Source: three-view drawing plus pictorial views. Frame: mm from the lowest corner of the part. A direction names the side the tool comes from. Coordinates: 2 decimals unless noted, no trailing zeros. Order: outer loops, then holes, each group sorted by start corner. A loop starts at its lowest first (then second) coordinate and runs counter-clockwise, first axis right, second up. Notation, with made-up numbers: M -27,35 L -18,35 A15 ccw -18,61 Z; hole C 8,31 d2. An arc over 180 degrees is marked long. One line per question, with ' | ' between items.
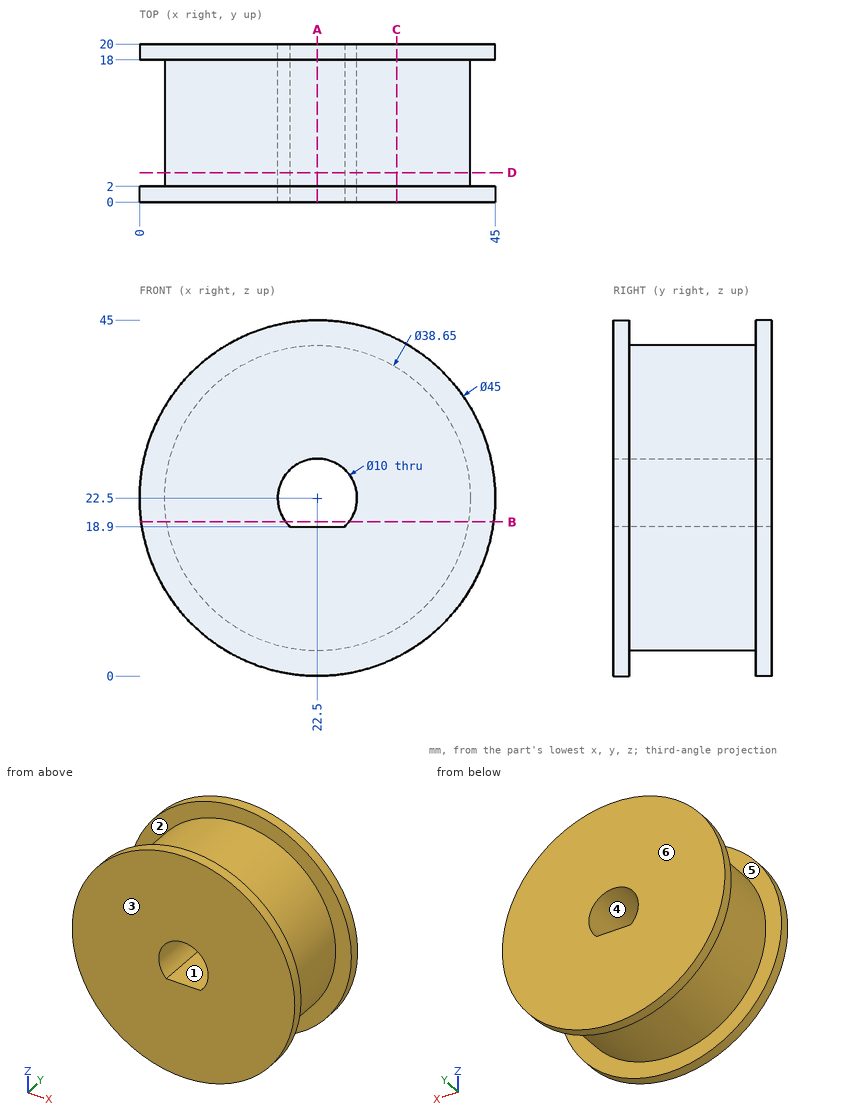
1. Access query for the marked faces 1 and 2. Directions: +Z, -Z, +X, -X, +Y, -Y. A direction counts if a zero-diameter tool reaches every point of the face in a straight line with its end or side. Return the directions, or none.
Response values:
face 1: +Y, -Y | face 2: none
2. Material intervals for line 1 (X direction, y = 11.5, z = 22.5) (3 decimals); line 2 (Z direction, x = 22.5, y = 5) (3 decimals); line 3 (Y direction, x = 22, z = 3), sorted ascending. Write a range as [from, to].
Response values:
line 1: x = [3.175, 17.5], [27.5, 41.825] | line 2: z = [3.175, 18.9], [27.5, 41.825] | line 3: y = [0, 2], [18, 20]
3. Section C-C, the plane x = 32.5. Output: boundary loops of the cut face in (y, z).
Response values:
outline: M 0,2.34 L 2,2.34 L 2,5.96 L 18,5.96 L 18,2.34 L 20,2.34 L 20,42.66 L 18,42.66 L 18,39.04 L 2,39.04 L 2,42.66 L 0,42.66 Z
4. Draft query along Y for the marked faces 3, 4, 5 and 6. Return one class per face: pulls with the +Y half, pulls with the -Y half, needs draft (parallel to the pull), parting line crosses it, or undercut.
Response values:
face 3: pulls with the -Y half | face 4: needs draft | face 5: undercut | face 6: pulls with the +Y half
5. Pin query (flat end, axial travel): P1, Ø10, axis at y = 7.5, z = 7.5, coming from the -X side; P2, Ø12, axis at x = 27.5, y = 5.5, coming from the -Z side; P3, Ø2, axis at x = 23, y = 5, coming from the +Z side (3 decimals); P4, Ø8, axis at x = 22.5, z = 22.5, coming from the +Y side. Return the tip coordinate at first contact, or that it passes through.
Response values:
P1: stops at x = 5.96 | P2: stops at z = 0 | P3: stops at z = 41.825 | P4: stops at y = 20
6. Section D-D, the plane y = 3.75. Output: boundary loops of the cut face in (x, z) (3 decimals).
Response values:
outline: C 22.5,22.5 d38.65; hole M 19.03,18.9 L 25.97,18.9 A5 ccw long Z
7. Section A-A, the plane x = 22.5. Output: boundary loops of the cut face in (y, z) (3 decimals).
Response values:
outline: M 0,0 L 2,0 L 2,3.175 L 18,3.175 L 18,0 L 20,0 L 20,18.9 L 0,18.9 Z; M 0,27.5 L 20,27.5 L 20,45 L 18,45 L 18,41.825 L 2,41.825 L 2,45 L 0,45 Z
8. Section B-B, the plane z = 19.5. Output: boundary loops of the cut face in (x, y).
Response values:
outline: M 0.2,0 L 18.5,0 L 18.5,20 L 0.2,20 L 0.2,18 L 3.41,18 L 3.41,2 L 0.2,2 Z; M 26.5,0 L 44.8,0 L 44.8,2 L 41.59,2 L 41.59,18 L 44.8,18 L 44.8,20 L 26.5,20 Z
